from build123d import *

# Parameters (mm, degrees)
AUFSATZ_LINEAR_AUSTRAGEN1_DEPTH = 25
SKIZZE2_W                       = 6
SKIZZE2_H                       = 1.8
AUFSATZ_LINEAR_AUSTRAGEN2_DEPTH = 8
SKIZZE3_W                       = 7.5
SKIZZE3_H                       = 0.15
SCHNITT_LINEAR_AUSTRAGEN1_DEPTH = 34
VERRUNDUNG1_R                   = 0.2


with BuildPart() as part:
    # Skizze1 → Aufsatz-Linear austragen1 (new body)
    with BuildSketch(Plane.XY):
        Polygon((-4.75, 0.9), (-6.7, 0.9), (-6.7, -0.9), (-4.75, -0.9), (-4.75, -2.9), (-3.75, -2.9), (-3.75, -0.9), (3.75, -0.9), (3.75, -2.9), (4.75, -2.9), (4.75, -0.9), (6.7, -0.9), (6.7, 0.9), (4.75, 0.9), (4.75, 2.9), (3.75, 2.9), (3.75, 0.9), (-3.75, 0.9), (-3.75, 2.9), (-4.75, 2.9), align=None)
    extrude(amount=AUFSATZ_LINEAR_AUSTRAGEN1_DEPTH)

    # Skizze2 → Aufsatz-Linear austragen2 (add)
    with BuildSketch(Plane(origin=(0, 0, 0), x_dir=(-1, 0, 0), z_dir=(0, 0, -1))):
        Rectangle(SKIZZE2_W, SKIZZE2_H)
    extrude(amount=AUFSATZ_LINEAR_AUSTRAGEN2_DEPTH)

    # Skizze3 → Schnitt-Linear austragen1 (cut, through all)
    with BuildSketch(Plane.XY.offset(25)):
        with Locations((0, -0.825)):
            Rectangle(SKIZZE3_W, SKIZZE3_H)
        with Locations((0, 0.825)):
            Rectangle(SKIZZE3_W, SKIZZE3_H)
    extrude(amount=-SCHNITT_LINEAR_AUSTRAGEN1_DEPTH, mode=Mode.SUBTRACT)

    # Verrundung1
    verrundung1_edges = [part.edges().sort_by_distance(p)[0] for p in [
        (0, 0.75, 25),
        (-4.75, -1.9, 25),
        (-4.25, -2.9, 25),
        (-5.725, 0.9, 0),
        (-4.75, 1.9, 0),
        (-4.25, 2.9, 0),
        (-3.75, -1.825, 25),
        (4.25, 2.9, 0),
        (4.75, 1.9, 0),
        (5.725, 0.9, 0),
        (6.7, 0, 0),
        (5.725, -0.9, 0),
        (4.75, -1.9, 0),
        (4.25, -2.9, 0),
        (-4.25, -2.9, 0),
        (-4.75, -1.9, 0),
        (-5.725, -0.9, 0),
        (-6.7, 0, 0),
        (3.75, -1.825, 25),
        (4.25, -2.9, 25),
        (-6.7, 0.9, 12.5),
        (-4.75, 2.9, 12.5),
        (-3.75, 2.9, 12.5),
        (3.75, 2.9, 12.5),
        (4.75, 2.9, 12.5),
        (6.7, 0.9, 12.5),
        (6.7, -0.9, 12.5),
        (4.75, -2.9, 12.5),
        (3.75, -2.9, 12.5),
        (-3.75, -2.9, 12.5),
        (-4.75, -2.9, 12.5),
        (-6.7, -0.9, 12.5),
        (4.75, -1.9, 25),
        (5.725, -0.9, 25),
        (6.7, 0, 25),
        (5.725, 0.9, 25),
        (-6.7, 0, 25),
        (4.75, 1.9, 25),
        (4.25, 2.9, 25),
        (3.75, 1.825, 25),
        (-3.75, 1.825, 25),
        (3, 0, -8),
        (-3, 0, -8),
        (-4.25, 2.9, 25),
        (0, 0.75, -8),
        (0, -0.75, -8),
        (-4.75, 1.9, 25),
        (-5.725, 0.9, 25),
        (0, -0.75, 25),
        (-5.725, -0.9, 25),
    ]]
    fillet(verrundung1_edges, radius=VERRUNDUNG1_R)


solid = part.part
Read the model definition and answer for the solid it produces. Units are mm, in the model's axes. A direction names the side the tool comes from. Round coordinates to 2 decimals unless told otherwise and drop trailing zeros. Write each loop counter-clockwise with the first axis right and the second up, starting at its lowest first coordinate (ties: lowest second). Pieces come first, ordered by that corner, then holes.
Q1. Find section D-D on y = 0. Determine the outline of the cut face in (x, z), and give its area (3 significant figures).
Values:
outline: (-6.7, 0.2) arc R0.2 ccw to (-6.5, 0) - (-3, 0) - (-3, -7.8) arc R0.2 ccw to (-2.8, -8) - (2.8, -8) arc R0.2 ccw to (3, -7.8) - (3, 0) - (6.5, 0) arc R0.2 ccw to (6.7, 0.2) - (6.7, 24.8) arc R0.2 ccw to (6.5, 25) - (-6.5, 25) arc R0.2 ccw to (-6.7, 24.8) - close
area: 383 mm2
Q2. Flat-ended cylindrical pins translate along their axes: P1, Ø1, axis at x = 5, y = 1, coming from the -Z side; P2, Ø1.6, axis at y = 0, z = -3.5, coming from the +X side; P3, Ø2, axis at x = 1, z = 3.5, coming from the -Y side. Find the tip coordinate at first contact, or state that the pin passes through.
Values:
P1: stops at z = 0
P2: stops at x = 3
P3: stops at y = -0.75
Q3. A tool of negligible diameter and unlimited length cuts with its end or side. For faces 5 (the face through (-3.75, -2, 13)), 6 (the face through (-3.75, 2, 12)), 7 (the face through (-4.75, 2, 12)), 8 (the face through (3, 0, -4)), from which of +Z, -Z, +X, -X, +Y, -Y can it reach the whole face along a straight path? Write none if from no direction.
Values:
face 5: +Z, -Z, -Y
face 6: +Z, -Z, +Y
face 7: +Z, -Z, -X, +Y
face 8: -Z, +X, +Y, -Y
Q4. Find section B-B on x = -0.75. Determine the outline of the cut face in (y, z).
Values:
outline: (-0.75, -7.8) arc R0.2 ccw to (-0.55, -8) - (0.55, -8) arc R0.2 ccw to (0.75, -7.8) - (0.75, 24.8) arc R0.2 ccw to (0.55, 25) - (-0.55, 25) arc R0.2 ccw to (-0.75, 24.8) - close
Q5. The mould has two halves that part along X. Classify faces 1 (the face through (6, -0.9, 12)), 2 (the face through (-3, 0, -4)), 3 (the face through (3.75, -2, 12)), 4 (the face through (4.75, -2, 12)): released by +X, released by -X, zero draft, split by the parting line, or undercut.
Values:
face 1: zero draft
face 2: released by -X
face 3: undercut
face 4: released by +X
Q6. Straight lines are drawn through the part: line 1 (X direction, y = 1.9, z = 15); line 2 (Z direction, x = -4.25, y = 0.5); line 3 (Y direction, x = 2, z = -0.5). For each, find the intervals that lie inside material, in ascending order.
Values:
line 1: x = -4.75 to -3.75, 3.75 to 4.75
line 2: z = 0 to 25
line 3: y = -0.75 to 0.75
Q7. Find section A-A on y = -1.6. Determine the outline of the cut face in (x, z), and give its area (3 significant figures).
Values:
outline: (-4.75, 0.2) arc R0.2 ccw to (-4.55, 0) - (-3.75, 0) - (-3.75, 24.8) arc R0.2 ccw to (-3.95, 25) - (-4.55, 25) arc R0.2 ccw to (-4.75, 24.8) - close; (3.75, 0) - (4.55, 0) arc R0.2 ccw to (4.75, 0.2) - (4.75, 24.8) arc R0.2 ccw to (4.55, 25) - (3.95, 25) arc R0.2 ccw to (3.75, 24.8) - close
area: 49.9 mm2
